```python
from build123d import *

# Parameters (mm, degrees)
CROQUIS2_R              = 1
SALIENTE_EXTRUIR1_DEPTH = 7
SALIENTE_EXTRUIR2_DEPTH = 3
CROQUIS4_R              = 2.5
CORTAR_EXTRUIR1_DEPTH   = 2.6
CROQUIS5_R              = 2.6
CORTAR_EXTRUIR3_DEPTH   = 2.2


with BuildPart() as part:
    # Croquis2 → Saliente-Extruir1 (new body)
    with BuildSketch(Plane(origin=(0, 0, 0), x_dir=(0, 0, -1), z_dir=(1, 0, 0))):
        with BuildLine():
            Line((-5, 0), (-5, 20))
            Line((-5, 20), (5, 20))
            Line((5, 20), (5, 0))
            ThreePointArc((5, 0), (0, -5), (-5, 0))
        make_face()
        Circle(CROQUIS2_R, mode=Mode.SUBTRACT)
    extrude(amount=SALIENTE_EXTRUIR1_DEPTH)

    # Croquis3 → Saliente-Extruir2 (add)
    with BuildSketch(Plane(origin=(0, 20, 0), x_dir=(1, 0, 0), z_dir=(0, 1, 0))):
        with BuildLine():
            Line((-27.897521221, -35), (42.102478779, -35))
            ThreePointArc((42.102478779, -35), (45.638012685, -33.535533906), (47.102478779, -30))
            Line((47.102478779, -30), (47.102478779, 30))
            ThreePointArc((47.102478779, 30), (45.638012685, 33.535533906), (42.102478779, 35))
            Line((42.102478779, 35), (-27.897521221, 35))
            ThreePointArc((-27.897521221, 35), (-31.433055127, 33.535533906), (-32.897521221, 30))
            Line((-32.897521221, 30), (-32.897521221, -30))
            ThreePointArc((-32.897521221, -30), (-31.433055127, -33.535533906), (-27.897521221, -35))
        make_face()
    extrude(amount=SALIENTE_EXTRUIR2_DEPTH)

    # Croquis4 → Cortar-Extruir1 (cut)
    with BuildSketch(Plane(origin=(7, 0, 0), x_dir=(0, 0, -1), z_dir=(1, 0, 0))):
        Circle(CROQUIS4_R)
    extrude(amount=-CORTAR_EXTRUIR1_DEPTH, mode=Mode.SUBTRACT)

    # Croquis5 → Cortar-Extruir3 (cut)
    with BuildSketch(Plane.ZY):
        Circle(CROQUIS5_R)
    extrude(amount=-CORTAR_EXTRUIR3_DEPTH, mode=Mode.SUBTRACT)


solid = part.part
```
The model under review builds one solid part; all positions refer to its coordinate system, in mm. A direction names the side the tool comes from. Round coordinates to 2 decimals unless told otherwise and drop trailing zeros. Order: outer loops, then holes, each group sorted by start corner. A loop starts at its lowest first (then second) coordinate and runs counter-clockwise, first axis right, second up. Notation, with made-up numbers: M -6.5,-24.5 L 19.5,-24.5 A12 ccw 19.5,-11.5 Z; hole C 37,16.5 d9. An arc over 180 degrees is marked long. Use a Markdown table: item, result.
1) Tool access review of faces 1 (the face through (3, 10, -5)), 2 (the face through (7, 8, 0)), 3 (the face through (4.4, -1, -1)), 4 (the face through (0, 8, 0)), 5 (the face through (3, 10, 5)): name each direction out of +Z, -Z, +X, -X, +Y, -Y from which nothing blocks a thin tool from reaching the whole face with its end or side.
Report:
| item | result |
|---|---|
| face 1 | -Z, +X, -X, -Y |
| face 2 | +Z, -Z, +X, -Y |
| face 3 | +X |
| face 4 | +Z, -Z, -X, -Y |
| face 5 | +Z, +X, -X, -Y |
2) Consider section B-B (y = 8.25). Write out the cut boundary in (x, z), then the cut area to 3 significant figures.
Report:
| item | result |
|---|---|
| outline | M 0,-5 L 7,-5 L 7,5 L 0,5 Z |
| area | 70.0 mm^2 |
3) Insertion check: pin 1 (3.5 mm diameter, centred on x = 4, y = 12, fed in from +Z); pin 2 (2.5 mm diameter, centred on y = 0, z = 0, fed in from -X); pin 3 (6 mm diameter, centred on y = 10, z = 5.5, fed in from +X). Each pin has a flat end and moves straight along its axis. Give the tip position at first contact, or say it passes through.
Report:
| item | result |
|---|---|
| pin 1 | z = 5 |
| pin 2 | x = 2.2 |
| pin 3 | x = 7 |
4) Wall thickness on line 1 along Z through (x, y) = (3.25, 0); line 2 along Y through (x, z) = (3.5, 0); line 3 along Y through (x, z) = (14, 5.5): over which ranges is each line inside the solid? List them lowest first. Write a range as [from, to].
Report:
| item | result |
|---|---|
| line 1 | [-5, -1], [1, 5] |
| line 2 | [-5, -1], [1, 23] |
| line 3 | [20, 23] |
5) Draft analysis for pull direction Y (two halves, no side actions). For faces 6 (the face through (45.677, 21.479, -33.496)), 7 (the face through (5.72, -2.44, 0.54)), 8 (the face through (3, -5, 0)), 9 (the face through (2.2, -1, 1)), state which applies: released by +Y, released by -Y, zero draft, split by the parting line, or undercut.
Report:
| item | result |
|---|---|
| face 6 | zero draft |
| face 7 | undercut |
| face 8 | released by -Y |
| face 9 | undercut |
6) Consider section C-C (x = -7.5). Write out the cut boundary in (y, z), then the cut area to 3 significant figures.
Report:
| item | result |
|---|---|
| outline | M 20,-35 L 23,-35 L 23,35 L 20,35 Z |
| area | 210 mm^2 |
7) Consider section A-A (z = 0). Write out the cut boundary in (x, y), then the cut area to 3 significant figures.
Report:
| item | result |
|---|---|
| outline | M -32.9,20 L 0,20 L 0,2.6 L 2.2,2.6 L 2.2,1 L 4.4,1 L 4.4,2.5 L 7,2.5 L 7,20 L 47.1,20 L 47.1,23 L -32.9,23 Z; M 0,-5 L 7,-5 L 7,-2.5 L 4.4,-2.5 L 4.4,-1 L 2.2,-1 L 2.2,-2.6 L 0,-2.6 Z |
| area | 386 mm^2 |
